Check sheet for the modelled part. Datum: model origin and axes. Units: mm. Give positions to 0.01 mm unless a question says otherwise; leave off trailing zeros. Loops run counter-clockwise (first coordinate to the right, second up) from the corner with the lowest first, then second, coordinate; pieces in that order, holes last. Notation, with made-up numbers: M 67,6 L 105,6 A10 ccw 105,13 Z; hole C -6.5,62.5 d2. An arc over 180 degrees is marked long. Use one line per item in the form item = value.
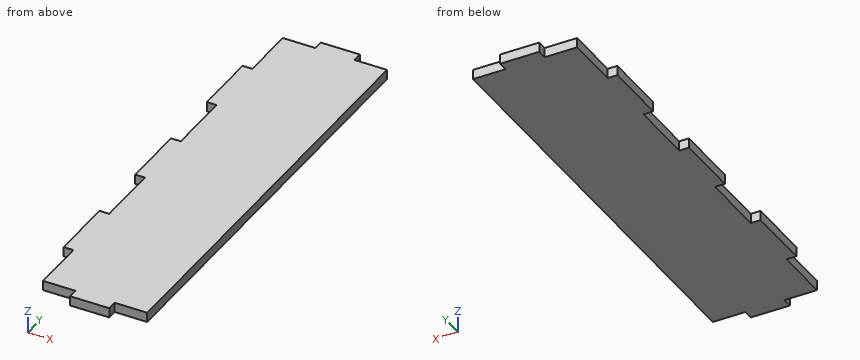
Autodesk Inventor part; units mm, degrees
ref_plane "YZ Plane" through (0, 0, 0) normal (1, 0, 0) x (0, 1, 0)
ref_plane "XZ Plane" through (0, 0, 0) normal (0, 1, 0) x (-1, 0, 0)
ref_plane "XY Plane" through (0, 0, 0) normal (0, 0, 1) x (1, 0, 0)
sketch "Sketch1" plane through (0, 0, 0) normal (0, 0, 1) x (1, 0, 0)
  line L0 (0, 0) -> (0, -20)
  line L1 (0, -20) -> (3, -20)
  line L2 (3, -20) -> (3, -37)
  line L3 (3, -37) -> (13, -37)
  line L4 (13, -37) -> (13, -40)
  line L5 (13, -40) -> (25, -40)
  line L6 (25, -40) -> (25, -37)
  line L7 (25, -37) -> (35, -37)
  line L8 (0, 0) -> (3, 0)
  line L9 (3, 0) -> (3, 20)
  line L10 (3, 20) -> (0, 20)
  line L11 (0, 20) -> (0, 30)
  line L12 (0, 30) -> (3, 30)
  line L13 (3, 30) -> (35, 30)
  line L14 (35, 30) -> (35, -37)
  dimension "d0" = 20
  dimension "d1" = 3
  dimension "d2" = 17
  dimension "d3" = 10
  dimension "d4" = 3
  dimension "d5" = 12
  dimension "d6" = 3
  dimension "d7" = 10
  dimension "d8" = 3
  dimension "d9" = 20
  dimension "d10" = 3
  dimension "d11" = 10
  dimension "d12" = 3
  dimension "d13" = 32
extrude "Extrusion1" add sketch "Sketch1" along normal blind 3
mirror "Mirror1" about plane through (35, 30, 0) normal (0, 1, 0) of "Extrusion1"
properties part number "voorkant"
1) Section check A-A (z = 1.95). Record the cut outline in (x, y), then the cut area to 3 significant figures.
Evaluation:
outline = M 0,-20 L 3,-20 L 3,-37 L 13,-37 L 13,-40 L 25,-40 L 25,-37 L 35,-37 L 35,97 L 25,97 L 25,100 L 13,100 L 13,97 L 3,97 L 3,80 L 0,80 L 0,60 L 3,60 L 3,40 L 0,40 L 0,20 L 3,20 L 3,0 L 0,0 Z
area = 4,540 mm^2
2) Section check C-C (x = 5). Record the cut outline in (y, z), then the cut area to 3 significant figures.
Evaluation:
outline = M -37,0 L 97,0 L 97,3 L -37,3 Z
area = 402 mm^2
3) Depth check by flat-ended pin: pin 1 Ø2 at (x, y) = (5.5, -2) entering from -Z; pin 2 Ø1.5 at (y, z) = (-24.5, 1) entering from -X; pin 3 Ø1.5 at (x, z) = (1.5, 1) entering from -Y; pin 4 Ø1.5 at (y, z) = (-38, 1.5) entering from +X. Enter the tip coordinate at first touch or a pass-through.
Evaluation:
pin_1 = 0
pin_2 = 3
pin_3 = -20
pin_4 = 25
4) Scan lines: line 1 (Y direction, x = 3.5, z = 2.4); line 2 (X direction, y = -27, z = 0.4). Record each from-to range of solid material in increasing order.
Evaluation:
line_1 = -37 to 97
line_2 = 3 to 35
5) Section check B-B (y = 45). Record the cut outline in (x, z), then the cut area to 3 significant figures.
Evaluation:
outline = M 3,0 L 35,0 L 35,3 L 3,3 Z
area = 96.0 mm^2
